from build123d import *

# Parameters (mm, degrees)
SKETCH7_W           = 40
SKETCH7_H           = 40
BOSS_EXTRUDE1_DEPTH = 11
LOFT1_START         = -20
LOFT1_DEPTH         = 40
SKETCH16_W          = 49.026286786
SKETCH16_H          = 65.242270374
SKETCH16_R          = 20
CUT_EXTRUDE3_DEPTH  = 6
SKETCH17_W          = 40
SKETCH17_H          = 5
BOSS_EXTRUDE5_DEPTH = 18
SKETCH10_R          = 2.25
CUT_EXTRUDE1_DEPTH  = 25
CHAMFER1_SIZE       = 2.5
FILLET3_R           = 20
SKETCH11_W          = 46.2
SKETCH11_H          = 14
BOSS_EXTRUDE6_DEPTH = 43
FILLET9_R           = 2.5
SKETCH20_W          = 40.6
SKETCH20_H          = 4.4
CUT_EXTRUDE4_DEPTH  = 40
SKETCH22_R          = 1.7
CUT_EXTRUDE5_DEPTH  = 30
FILLET11_R          = 2
CUT_EXTRUDE6_DEPTH  = 4
SKETCH24_R          = 3
CUT_EXTRUDE7_DEPTH  = 3


# Read off the part's stored shape, not the designer's step: Loft1
with BuildPart() as part:
    # Sketch7 → Boss-Extrude1 (new body)
    with BuildSketch(Plane.XY):
        Rectangle(SKETCH7_W, SKETCH7_H)
    extrude(amount=BOSS_EXTRUDE1_DEPTH)

    # Loft1 outline → Loft1 (add)
    with BuildSketch(Plane.YZ.offset(LOFT1_START)):
        with BuildLine():
            add(Edge.make_bspline(
                [(-38, 16), (-31.772819436, 16), (-26.227180564, 11), (-20, 11)],
                knots=[0, 0, 0, 0, 1, 1, 1, 1], degree=3))
            Line((-38, 16), (-38, 11))
            add(Edge.make_bspline(
                [(-38, 11), (-31.772819436, 11), (-26.227180564, 6), (-20, 6)],
                knots=[0, 0, 0, 0, 1, 1, 1, 1], degree=3))
            Line((-20, 6), (-20, 11))
        make_face()
    extrude(amount=LOFT1_DEPTH)

    # Sketch16 → Cut-Extrude3 (cut)
    with BuildSketch(Plane(origin=(0, 0, 0), x_dir=(-1, 0, 0), z_dir=(0, 0, -1))):
        Rectangle(SKETCH16_W, SKETCH16_H)
        Circle(SKETCH16_R, mode=Mode.SUBTRACT)
    extrude(amount=-CUT_EXTRUDE3_DEPTH, mode=Mode.SUBTRACT)

    # Sketch17 → Boss-Extrude5 (add)
    with BuildSketch(Plane(origin=(0, -38, 0), x_dir=(-1, 0, 0), z_dir=(0, -1, 0))):
        with Locations((0, -13.5)):
            Rectangle(SKETCH17_W, SKETCH17_H)
    extrude(amount=BOSS_EXTRUDE5_DEPTH)

    # Sketch10 → Cut-Extrude1 (cut)
    with BuildSketch(Plane.XY.offset(11)):
        with Locations((-7.00009521, 12.124420806)):
            Circle(SKETCH10_R)
        with Locations((6.99990479, 12.124420806)):
            Circle(SKETCH10_R)
        with Locations((13.99990479, 6.5153e-05)):
            Circle(SKETCH10_R)
        with Locations((6.99990479, -12.1242905)):
            Circle(SKETCH10_R)
        with Locations((-7.00009521, -12.1242905)):
            Circle(SKETCH10_R)
        with Locations((-14.00009521, 6.5153e-05)):
            Circle(SKETCH10_R)
    extrude(amount=-CUT_EXTRUDE1_DEPTH, mode=Mode.SUBTRACT)

    # Chamfer1
    chamfer1_edges = [part.edges().sort_by_distance(p)[0] for p in [
        (4.74990479, 12.124420806, 11),
        (-9.25009521, 12.124420806, 11),
        (-16.25009521, 6.5153e-05, 11),
        (-9.25009521, -12.1242905, 11),
        (4.74990479, -12.1242905, 11),
        (11.74990479, 6.5153e-05, 11),
    ]]
    chamfer(chamfer1_edges, length=CHAMFER1_SIZE)

    # Fillet3
    fillet3_edges = [part.edges().sort_by_distance(p)[0] for p in [
        (20, 20, 8.5),
        (-20, 20, 8.5),
    ]]
    fillet(fillet3_edges, radius=FILLET3_R - 0.0001)  # a hair under: the kernel refuses the full size

    # Sketch11 → Boss-Extrude6 (add)
    with BuildSketch(Plane(origin=(0, -56, -3.472963553), x_dir=(1, 0, 0), z_dir=(0, 1, 0))):
        with Locations((0, -12.472963553)):
            Rectangle(SKETCH11_W, SKETCH11_H)
    extrude(amount=-BOSS_EXTRUDE6_DEPTH)

    # Fillet9
    fillet9_edges = [part.edges().sort_by_distance(p)[0] for p in [
        (0, -56, 11),
        (-20, -56, 13.5),
        (20, -56, 13.5),
    ]]
    fillet(fillet9_edges, radius=FILLET9_R)

    # Sketch20 → Cut-Extrude4 (cut)
    with BuildSketch(Plane.XZ.offset(99)):
        with Locations((0, 9)):
            Rectangle(SKETCH20_W, SKETCH20_H)
    extrude(amount=-CUT_EXTRUDE4_DEPTH, mode=Mode.SUBTRACT)

    # Sketch22 → Cut-Extrude5 (cut)
    with BuildSketch(Plane.XY):
        with Locations(Location((11, -68.5, 0), (0, 0, 180))):
            Circle(SKETCH22_R)
        with Locations(Location((11, -90.5, 0), (0, 0, 180))):
            Circle(SKETCH22_R)
        with Locations(Location((-11, -90.5, 0), (0, 0, 180))):
            Circle(SKETCH22_R)
        with Locations(Location((-11, -68.5, 0), (0, 0, 180))):
            Circle(SKETCH22_R)
    extrude(amount=CUT_EXTRUDE5_DEPTH, mode=Mode.SUBTRACT)

    # Fillet11
    fillet11_edges = [part.edges().sort_by_distance(p)[0] for p in [
        (-23.1, -77.5, 16),
        (-23.1, -77.5, 2),
        (23.1, -77.5, 16),
        (23.1, -77.5, 2),
    ]]
    fillet(fillet11_edges, radius=FILLET11_R)

    # Sketch23 → Cut-Extrude6 (cut)
    with BuildSketch(Plane.XY.offset(16)):
        Polygon((-11, -65.324573519), (-13.75, -66.91228676), (-13.75, -70.08771324), (-11, -71.675426481), (-8.25, -70.08771324), (-8.25, -66.91228676), align=None)
        Polygon((11, -65.324573519), (8.25, -66.91228676), (8.25, -70.08771324), (11, -71.675426481), (13.75, -70.08771324), (13.75, -66.91228676), align=None)
        Polygon((11, -87.324573519), (8.25, -88.91228676), (8.25, -92.08771324), (11, -93.675426481), (13.75, -92.08771324), (13.75, -88.91228676), align=None)
        Polygon((-11, -87.324573519), (-13.75, -88.91228676), (-13.75, -92.08771324), (-11, -93.675426481), (-8.25, -92.08771324), (-8.25, -88.91228676), align=None)
    extrude(amount=-CUT_EXTRUDE6_DEPTH, mode=Mode.SUBTRACT)

    # Sketch24 → Cut-Extrude7 (cut)
    with BuildSketch(Plane(origin=(0, 0, 2), x_dir=(-1, 0, 0), z_dir=(0, 0, -1))):
        with Locations((-11, -68.5)):
            Circle(SKETCH24_R)
        with Locations((11, -68.5)):
            Circle(SKETCH24_R)
        with Locations((11, -90.5)):
            Circle(SKETCH24_R)
        with Locations((-11, -90.5)):
            Circle(SKETCH24_R)
    extrude(amount=-CUT_EXTRUDE7_DEPTH, mode=Mode.SUBTRACT)


solid = part.part
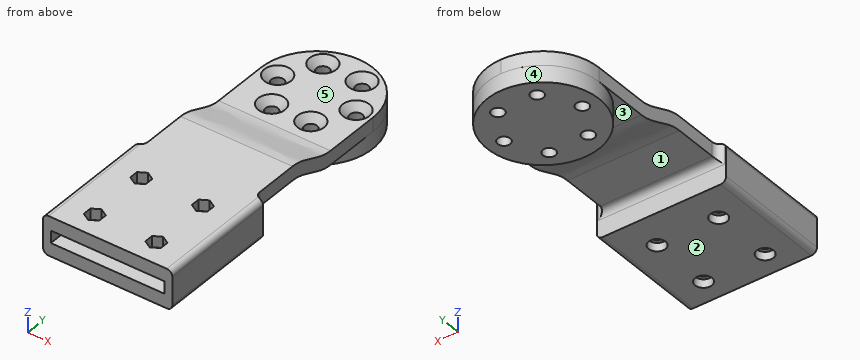
Model file for the job. Use its own axes, mm. Face numbers are marked on the shaded views. A direction names the side the tool comes from. Coordinates: 2 decimals unless noted, no trailing zeros. Write each loop counter-clockwise with the first axis right and the second up, starting at its lowest first coordinate (ties: lowest second). Pieces come first, ordered by that corner, then holes. Notation, with made-up numbers: (-31, -32.75) - (-18, -32.75) arc R25 ccw to (-18, -10.75) - close; hole circle Ø2 at (32.25, 75.5). An arc over 180 degrees is marked (long way). Write each question's results on one line, items separated by ' | '. Start each with the question number.
1) Probe line 1 along X through (y, z) = (-90.5, 5.55); line 2 along Z through (x, y) = (6, -91.5); line 3 along X through (y, z) = (-91, 10.25). List the from-to ranges inside material, lowest first. Write a range as from..to.
2) Cut at A-A (y = -78). Write the cut outline in (x, z), then the cut area to 3 significant figures.
3) Flat gauge pins, fed straight in: P1, Ø8, axis at x = 10.5, z = 7, coming from the +Y side; P2, Ø1, axis at x = -13, y = -74, coming from the -Z side; P3, Ø5.5, axis at x = -11, y = -68.5, coming from the -Z side; P4, Ø5, axis at x = 7, y = -12.12, coming from the -Z side. Where does each tip first touch, or does it go through?
4) 3-axis set-ups, long thin cutter, end or side, ignore diameter. For the marked faces 1, 2, 3, 4 and 5: which of +Z, -Z, +X, -X, +Y, -Y reach the whole face in a straight line?
5) Cut at B-B (y = -90.5). Count the separate pieces of the cut face and the enclosed holes in it, then the cut area to 3 significant figures.
6) Cut at C-C (y = -45). Write the cut outline in (x, z), then the cut area to 3 significant figures.
Returned:
1) line 1: -23.1..-12.7, -9.3..9.3, 12.7..23.1 | line 2: 2..6.8, 11.2..16 | line 3: -23.1..-20.3, 20.3..23.1
2) outline: (-23.1, 4) arc R2 ccw to (-21.1, 2) - (21.1, 2) arc R2 ccw to (23.1, 4) - (23.1, 14) arc R2 ccw to (21.1, 16) - (-21.1, 16) arc R2 ccw to (-23.1, 14) - close; hole (-20.3, 6.8) - (20.3, 6.8) - (20.3, 11.2) - (-20.3, 11.2) - close | area: 465 mm^2
3) P1: y = 18.91 | P2: z = 2 | P3: z = 5 | P4: z = 0
4) face 1: -Z, +X, -X | face 2: -Z, +X, -X, -Y | face 3: -Z, -X | face 4: -Z | face 5: +Z, +X, -X, +Y
5) separate pieces: 4 | enclosed holes: 0 | area: 367 mm^2
6) outline: (-20, 11) - (20, 11) - (20, 16) - (-20, 16) - close | area: 200 mm^2
